Verification items for this drawing (mm, ordinates from the low corner). A direction names the side the tool comes from. Coordinates: 2 decimals unless noted, no trailing zeros. Loops run counter-clockwise (first coordinate to the right, second up) from the corner with the lowest first, then second, coordinate; pieces in that order, holes last. Notation, with made-up numbers: M 29,82 L 56,82 A18 cw 56,88 Z; hole C 27,11.5 d9. An arc over 180 degrees is marked long. One line per question, with ' | ' between items. Start each with the question number.
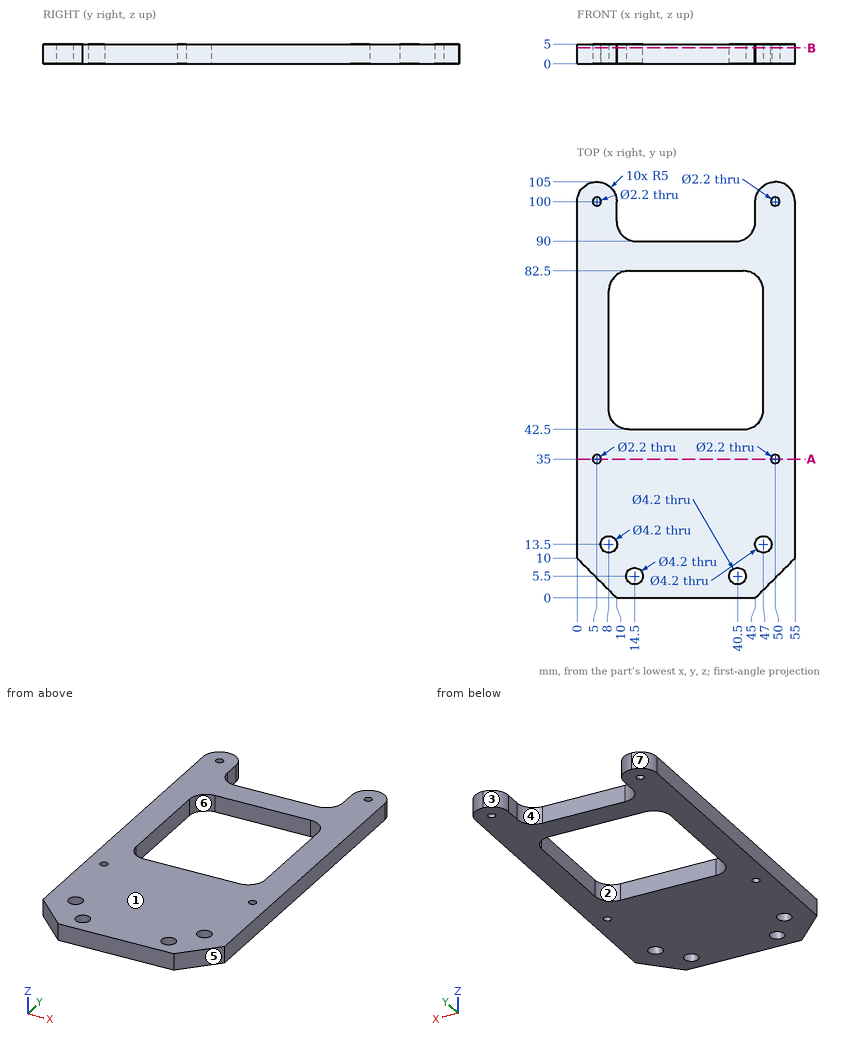
1. Tool access check on the marked faces 1, 2 and 3. Record the directions out of +Z, -Z, +X, -X, +Y, -Y that give a thin tool (end or side, any length) a straight path to the whole face; none if there is none.
2. Draft check along X on the marked faces 4, 5, 6 and 7. Enter one of: +X half, -X half, draft (parallel to the pull), parting line (faces both ways), or undercut.
3. Sectioned sample at A-A (y = 35). Record the cut outline in (x, z).
4. Thickness scan on line 1 (Y direction, x = 5, z = 2.85); line 2 (X direction, y = 100, z = 2.35); line 3 (Y direction, x = 34, z = 1.45). Record the ranges inside material, lowest first.
5. Depth check by flat-ended pin: pin 1 Ø1.3 at (x, y) = (50, 100) entering from -Z. Enter the tip coordinate at first touch or a pass-through.
6. Sectioned sample at B-B (z = 4). State how many separate pieces and enclosed holes the cut face has, and give its area (3 significant figures).
Result:
1) face 1: +Z, +X, -X, +Y, -Y | face 2: +Z, -Z | face 3: +Z, -Z, +Y
2) face 4: undercut | face 5: +X half | face 6: undercut | face 7: -X half
3) outline: M 0,0 L 3.9,0 L 3.9,5 L 0,5 Z; M 6.1,0 L 48.9,0 L 48.9,5 L 6.1,5 Z; M 51.1,0 L 55,0 L 55,5 L 51.1,5 Z
4) line 1: y = 5 to 33.9, 36.1 to 98.9, 101.1 to 105 | line 2: x = 0 to 3.9, 6.1 to 10, 45 to 48.9, 51.1 to 55 | line 3: y = 0 to 42.5, 82.5 to 90
5) pin 1: passes through
6) separate pieces: 1 | enclosed holes: 9 | area: 3,530 mm2
